Source: CAD feature listing. Evaluate the final solid. Frame: model axes, mm. Face numbers are marked on the shaded views. A direction names the side the tool comes from. Round coordinates to 2 decimals unless told otherwise and drop trailing zeros. Loops run counter-clockwise (first coordinate to the right, second up) from the corner with the lowest first, then second, coordinate; pieces in that order, holes last. Notation, with made-up numbers: (56.25, -39.5) -> (92.25, -39.5) arc R35 ccw to (92.25, -4.5) -> close; hole circle Ø4 at (80.25, -9.75). An arc over 180 degrees is marked (long way). Put each result on its own line as item: value. Start each with the question number.
1. Contact query for flat-ended pins moving along their axis: pin 1 (7.5 mm diameter, centred on x = 0, z = 12, fed in from +Y); pin 2 (2.5 mm diameter, centred on x = -8, y = -6, fed in from +Z); pin 3 (1.5 mm diameter, centred on x = -10, z = 9, fed in from -Y). Output: stop coordinate, or through.
2. Material intervals for L1, parallel to X at y = 23.5, z = 6.25; L2, parallel to X at y = 1, z = 16.5; L3, parallel to Y at x = 7.5, z = 5.25, sorted ascending.
3. Cut plane D-D (x = 3). Return the cut outline in (y, z), then the cut area to 3 significant figures.
4. Draft query along X for the marked faces 1, 2 and 3. Return one class per face: pulls with the +X half, pulls with the -X half, needs draft (parallel to the pull), parting line crosses it, or undercut.
5. Cut plane B-B (x = -8). Return the cut outline in (y, z), then the cut area to 3 significant figures.
6. Cut plane C-C (z = 12.5). Return the cut outline in (x, y), then the cut area to 3 significant figures.
7. Cut plane A-A (y = 6). Return the cut outline in (x, z).
8. Set-up query: the marked faces 4, 5 and 6. Return all of +Z, -Z, +X, -X, +Y, -Y with unobstructed straight access to the full face (end or side cutting, diameter ignored); none if empty.
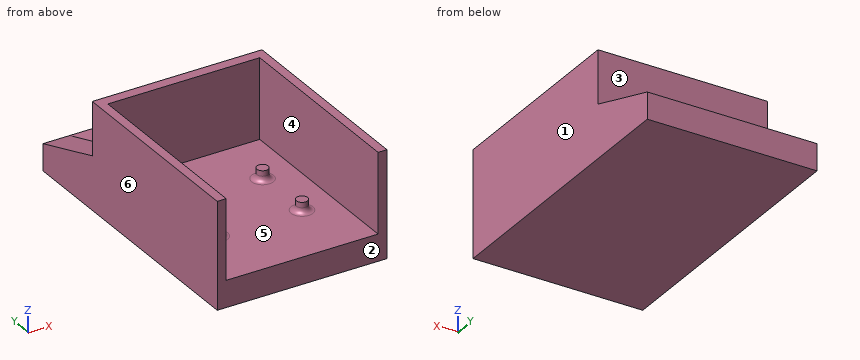
```python
from build123d import *

# Parameters (mm, degrees)
SKETCH_1_W      = 31.852941176
SKETCH_1_H      = 38
EXTRUDE_1_DEPTH = 5
EXTRUDE_2_DEPTH = 15
SKETCH_3_R      = 1.05
EXTRUDE_3_DEPTH = 2
SKETCH_4_W      = 31.852941176
SKETCH_4_H      = 15
EXTRUDE_4_DEPTH = 5
EXTRUDE_5_DEPTH = 5
EXTRUDE_6_DEPTH = 5
FILLET_1_R      = 1


with BuildPart() as part:
    # 草图1 → 凸台-拉伸1 (new body)
    with BuildSketch(Plane.XY):
        Rectangle(SKETCH_1_W, SKETCH_1_H)
    extrude(amount=EXTRUDE_1_DEPTH)

    # 草图2 → 凸台-拉伸2 (add)
    with BuildSketch(Plane.XY.offset(5)):
        Polygon((-14.25, -19), (-14.25, -17), (-14.25, 17), (14.25, 17), (14.25, -17), (14.25, -19), (15.926470588, -19), (15.926470588, 19), (-15.926470588, 19), (-15.926470588, -19), align=None)
    extrude(amount=EXTRUDE_2_DEPTH)

    # 草图3 → 凸台-拉伸3 (add)
    with BuildSketch(Plane.XY.offset(5)):
        with Locations((-8, 6)):
            Circle(SKETCH_3_R)
        with Locations((8, 6)):
            Circle(SKETCH_3_R)
        with Locations((-8, -6)):
            Circle(SKETCH_3_R)
        with Locations((8, -6)):
            Circle(SKETCH_3_R)
    extrude(amount=EXTRUDE_3_DEPTH)

    # 草图4 → 凸台-拉伸4 (add)
    with BuildSketch(Plane(origin=(0, 0, 0), x_dir=(-1, 0, 0), z_dir=(0, 0, -1))):
        with Locations((0, 26.5)):
            Rectangle(SKETCH_4_W, SKETCH_4_H)
    extrude(amount=-EXTRUDE_4_DEPTH)

    # 草图5 → 凸台-拉伸5 (add)
    with BuildSketch(Plane.ZY.offset(15.926470588)):
        Polygon((5, 34), (10, 19), (5, 19), align=None)
    extrude(amount=-EXTRUDE_5_DEPTH)

    # 草图6 → 凸台-拉伸6 (add)
    with BuildSketch(Plane(origin=(15.926470588, 0, 0), x_dir=(0, 0, -1), z_dir=(1, 0, 0))):
        Polygon((-5, 19), (-5, 34), (-10, 19), align=None)
    extrude(amount=-EXTRUDE_6_DEPTH)

    # 圆角1
    fillet_1_edges = [part.edges().sort_by_distance(p)[0] for p in [
        (-9.05, 6, 5),
        (6.95, 6, 5),
        (-9.05, -6, 5),
        (6.95, -6, 5),
    ]]
    fillet(fillet_1_edges, radius=FILLET_1_R)


solid = part.part
```
Solution:
1. pin 1: stops at y = 19
1. pin 2: stops at z = 7
1. pin 3: stops at y = 17
2. L1: x = -15.93 to -10.93, 10.93 to 15.93
2. L2: x = -15.93 to -14.25, 14.25 to 15.93
2. L3: y = -7.3 to -4.7, 4.7 to 7.3, 17 to 19
3. outline: (-19, 0) -> (34, 0) -> (34, 5) -> (19, 5) -> (19, 20) -> (17, 20) -> (17, 5) -> (-19, 5) -> close
3. area: 295 mm^2
4. face 1: pulls with the +X half
4. face 2: needs draft
4. face 3: undercut
5. outline: (-19, 0) -> (34, 0) -> (34, 5) -> (19, 5) -> (19, 20) -> (17, 20) -> (17, 5) -> (8.05, 5) arc R1 cw to (7.05, 6) -> (7.05, 7) -> (4.95, 7) -> (4.95, 6) arc R1 cw to (3.95, 5) -> (-3.95, 5) arc R1 cw to (-4.95, 6) -> (-4.95, 7) -> (-7.05, 7) -> (-7.05, 6) arc R1 cw to (-8.05, 5) -> (-19, 5) -> close
5. area: 304 mm^2
6. outline: (-15.93, -19) -> (-14.25, -19) -> (-14.25, 17) -> (14.25, 17) -> (14.25, -19) -> (15.93, -19) -> (15.93, 19) -> (-15.93, 19) -> close
6. area: 184 mm^2
7. outline: (-15.93, 0) -> (15.93, 0) -> (15.93, 20) -> (14.25, 20) -> (14.25, 5) -> (10.05, 5) arc R1 cw to (9.05, 6) -> (9.05, 7) -> (6.95, 7) -> (6.95, 6) arc R1 cw to (5.95, 5) -> (-5.95, 5) arc R1 cw to (-6.95, 6) -> (-6.95, 7) -> (-9.05, 7) -> (-9.05, 6) arc R1 cw to (-10.05, 5) -> (-14.25, 5) -> (-14.25, 20) -> (-15.93, 20) -> close
8. face 4: +Z, -Y
8. face 5: +Z
8. face 6: +Z, -Z, -X, +Y, -Y
